from build123d import *

# Parameters (mm, degrees)
SKETCH_1_R          = 42.5
EXTRUDE_1_DEPTH     = 20
SKETCH_2_R          = 15
EXTRUDE_2_DEPTH     = 4
SKETCH_3_R          = 38
CUT_EXTRUDE_1_DEPTH = 13
SKETCH_4_R          = 11
CUT_EXTRUDE_2_DEPTH = 20
SKETCH_5_R          = 3.25
CUT_EXTRUDE_3_DEPTH = 20
SKETCH_6_R          = 6
CUT_EXTRUDE_4_DEPTH = 4
SKETCH_8_R          = 1.5
CUT_EXTRUDE_5_DEPTH = 100
SKETCH_9_R          = 1.5
CUT_EXTRUDE_6_DEPTH = 100
CUT_EXTRUDE_7_DEPTH = 13


with BuildPart() as part:
    # ｽｹｯﾁ1 → ﾎﾞｽ - 押し出し1 (new body)
    with BuildSketch(Plane(origin=(0, 0, 0), x_dir=(1, 0, 0), z_dir=(0, 1, 0))):
        Circle(SKETCH_1_R)
    extrude(amount=EXTRUDE_1_DEPTH)

    # ｽｹｯﾁ2 → ﾎﾞｽ - 押し出し2 (add)
    with BuildSketch(Plane(origin=(0, 20, 0), x_dir=(1, 0, 0), z_dir=(0, 1, 0))):
        Circle(SKETCH_2_R)
    extrude(amount=EXTRUDE_2_DEPTH)

    # ｽｹｯﾁ3 → ｶｯﾄ - 押し出し1 (cut)
    with BuildSketch(Plane.XZ):
        Circle(SKETCH_3_R)
    extrude(amount=-CUT_EXTRUDE_1_DEPTH, mode=Mode.SUBTRACT)

    # ｽｹｯﾁ4 → ｶｯﾄ - 押し出し2 (cut)
    with BuildSketch(Plane(origin=(0, 24, 0), x_dir=(1, 0, 0), z_dir=(0, 1, 0))):
        Circle(SKETCH_4_R)
    extrude(amount=-CUT_EXTRUDE_2_DEPTH, mode=Mode.SUBTRACT)

    # ｽｹｯﾁ5 → ｶｯﾄ - 押し出し3 (cut)
    with BuildSketch(Plane(origin=(0, 20, 0), x_dir=(1, 0, 0), z_dir=(0, 1, 0))):
        with Locations((25, 0)):
            Circle(SKETCH_5_R)
        with Locations((0, -25)):
            Circle(SKETCH_5_R)
        with Locations((-25, 0)):
            Circle(SKETCH_5_R)
        with Locations((0, 25)):
            Circle(SKETCH_5_R)
    extrude(amount=-CUT_EXTRUDE_3_DEPTH, mode=Mode.SUBTRACT)

    # ｽｹｯﾁ6 → ｶｯﾄ - 押し出し4 (cut)
    with BuildSketch(Plane.XZ.offset(-13)):
        with Locations((25, 0)):
            Circle(SKETCH_6_R)
        with Locations((0, -25)):
            Circle(SKETCH_6_R)
        with Locations((-25, 0)):
            Circle(SKETCH_6_R)
        with Locations((0, 25)):
            Circle(SKETCH_6_R)
    extrude(amount=-CUT_EXTRUDE_4_DEPTH, mode=Mode.SUBTRACT)

    # ｽｹｯﾁ8 → ｶｯﾄ - 押し出し5 (cut)
    with BuildSketch(Plane(origin=(30.0520382, 0, 30.0520382), x_dir=(-0.707106781, 0, 0.707106781), z_dir=(-0.707106781, 0, -0.707106781))):
        with Locations((0, 5)):
            Circle(SKETCH_8_R)
    extrude(amount=CUT_EXTRUDE_5_DEPTH, mode=Mode.SUBTRACT)

    # ｽｹｯﾁ9 → ｶｯﾄ - 押し出し6 (cut)
    with BuildSketch(Plane(origin=(-30.0520382, 0, 30.0520382), x_dir=(0.707106781, 0, 0.707106781), z_dir=(-0.707106781, 0, 0.707106781))):
        with Locations((0, 5)):
            Circle(SKETCH_9_R)
    extrude(amount=-CUT_EXTRUDE_6_DEPTH, mode=Mode.SUBTRACT)

    # ｽｹｯﾁ10 → ｶｯﾄ - 押し出し7 (cut)
    with BuildSketch(Plane(origin=(0, 0, 0), x_dir=(-1, 0, 0), z_dir=(0, -1, 0))):
        Polygon((25.102290732, 34.294678888), (-34.294678888, -25.102290732), (-41.012193309, -18.384776311), (18.384776311, 41.012193309), align=None)
    extrude(amount=-CUT_EXTRUDE_7_DEPTH, mode=Mode.SUBTRACT)


solid = part.part
CAD build for the part. Positions are in the model's coordinates, mm. A direction names the side the tool comes from. Coordinates: 2 decimals unless noted, no trailing zeros. Order: outer loops, then holes, each group sorted by start corner. A loop starts at its lowest first (then second) coordinate and runs counter-clockwise, first axis right, second up.
Item 1: Band-saw the part on D-D on y = 15.5. List the corners of the cut face in (x, z), plus the area to 3 significant figures.
Check sheet entries:
outline: circle Ø85 at (0, 0); hole circle Ø12 at (-25, 0); hole circle Ø22 at (0, 0); hole circle Ø12 at (0, -25); hole circle Ø12 at (0, 25); hole circle Ø12 at (25, 0)
area: 4,840 mm2
Item 2: Drill centre lines: L1, parallel to X at y = 18.05, z = 0; L2, parallel to Z at x = -5.5, y = 16; L3, parallel to X at y = 8.5, z = 0. Where is each one in solid material? Low to high.
Check sheet entries:
L1: x = -42.5 to -28.25, -21.75 to -11, 11 to 21.75, 28.25 to 42.5
L2: z = -42.14 to -27.4, -22.6 to -9.53, 9.53 to 22.6, 27.4 to 42.14
L3: x = -42.5 to -38, 38 to 42.5
Item 3: Pin check, flat tips, straight feed: pin 1 Ø19 at (x, z) = (0, -25) entering from -Y; pin 2 Ø10 at (y, z) = (2.5, 23.5) entering from -X; pin 3 Ø19 at (x, z) = (0, 25) entering from +Y. Stop position of each tip, or through.
Check sheet entries:
pin 1: stops at y = 13
pin 2: stops at x = -38.26
pin 3: stops at y = 20
Item 4: Band-saw the part on A-A on y = 8. List the corners of the cut face in (x, z), plus the area to 3 significant figures.
Check sheet entries:
outline: (-25.1, -34.29) - (-21.88, -31.07) arc R38 cw (long way) to (31.07, 21.88) - (34.29, 25.1) arc R42.5 ccw (long way) to start; (-16.53, -39.15) arc R42.5 ccw to (39.15, 16.53) - (35.69, 13.06) arc R38 cw to (-13.06, -35.69) - close
area: 1,050 mm2
Item 5: Band-saw the part on B-B on x = 0. Give the number of separate pieces and of enclosed holes in the cut face, plus the area to 3 significant figures.
Check sheet entries:
separate pieces: 4
enclosed holes: 0
area: 455 mm2
Item 6: Two-plate mould, pull along Y, no slides. Class faces 6 (the face through (-2.38, 18.58, 10.74)), 7 (the face through (-27.49, 4.43, 29.45)), 8 (the face through (-5, 24, -10)): +Y half, -Y half, draft (parallel to the pull), parting line (faces both ways), or undercut.
Check sheet entries:
face 6: draft
face 7: undercut
face 8: +Y half
Item 7: 3-axis set-ups, long thin cutter, end or side, ignore diameter. For faces 1 (the face through (-22, 17, -3)), 2 (the face through (-27.646, 6.014, -29.21)), 3 (the face through (-14.985, 21.972, -0.66)), 4 (the face through (37.445, 6.409, 14.817)), 5 (the face through (21.753, 18.521, -0.143)): which of +Z, -Z, +X, -X, +Y, -Y reach the whole face in a straight line?
Check sheet entries:
face 1: -Y
face 2: none
face 3: +Y
face 4: +Z, -Y
face 5: +Y, -Y
